Can you work these out from the model? Positions are in its coordinate system, mm. Round coordinates to 2 decimals unless told otherwise and drop trailing zeros. Order: outer loops, then holes, each group sorted by start corner. A loop starts at its lowest first (then second) coordinate and runs counter-clockwise, first axis right, second up. Notation, with made-up numbers: (83.25, -21) -> (115.25, -21) arc R20 ccw to (115.25, -16) -> close; hole circle Ø8 at (45, 1). An arc over 180 degrees is marked (long way). One line per item, written item: value.
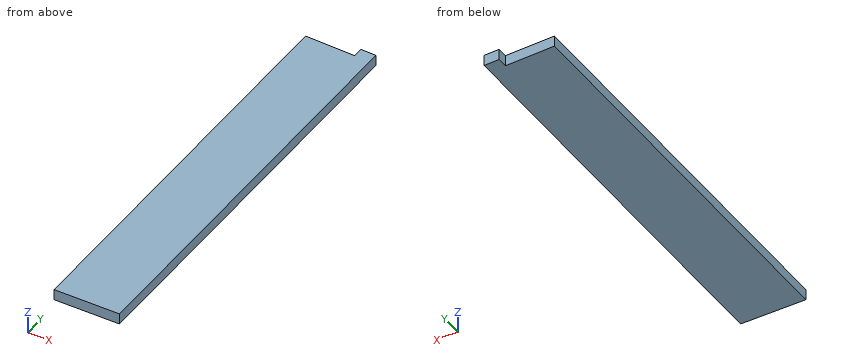
Autodesk Inventor part; units mm, degrees
ref_plane "YZ Plane" through (0, 0, 0) normal (1, 0, 0) x (0, 1, 0)
ref_plane "XZ Plane" through (0, 0, 0) normal (0, 1, 0) x (-1, 0, 0)
ref_plane "XY Plane" through (0, 0, 0) normal (0, 0, 1) x (1, 0, 0)
sketch "Sketch1" plane through (0, 0, 0) normal (0, 0, 1) x (1, 0, 0)
  line L0 (65.4735, 181.5397) -> (65.4735, -8.4603)
  line L1 (65.4735, -8.4603) -> (95.4735, -8.4603)
  line L2 (95.4735, -8.4603) -> (95.4735, 180.4921)
  line L3 (65.4735, 181.5397) -> (95.4735, 180.4921)
  line L4 (65.4735, 181.5397) -> (99.7821, 181.5397) construction
  line L5 (95.4735, 180.4921) -> (95.4735, 185.4921)
  line L6 (95.4735, 185.4921) -> (88.4735, 185.4921)
  line L7 (88.4735, 185.4921) -> (88.4735, 180.7366)
  line L8 (88.4735, 185.4921) -> (98.5031, 185.1419)
  line L9 (88.4735, 185.4921) -> (98.5092, 185.4921) construction
  point P0 (0, 0)
  point P1 (95.4735, 185.2477)
  dimension "d0" = 190
  dimension "d1" = 30
  dimension "d2" = 2
  dimension "d4" = 7
  dimension "d6" = 2
  dimension "d12" = 5
extrude "Extrusion1" add sketch "Sketch1" along normal blind 5 contours L3 L2 L1 L0 | L7 L8 L5 L3
properties part number "protostand"
Q1. Please list where these lines run through material, in increasing order: line 1 along Y through (x, z) = (88, 2.35); line 2 along Y through (x, z) = (79.5, 4.2).
Answers below:
line 1: -8.46 to 180.75
line 2: -8.46 to 181.05
Q2. I want a section at A-A on z = 1.2. List the corners of the cut face in (x, y) for me.
Answers below:
outline: (65.47, -8.46) -> (95.47, -8.46) -> (95.47, 185.25) -> (88.47, 185.49) -> (88.47, 180.74) -> (65.47, 181.54) -> close
Q3. Will this pin go through, and if not, where does the flat tip stop? pin 1 Ø8 at (x, y) = (78.5, 12) entering from -Z.
Answers below:
pin 1: z = 0
Q4. I want a section at C-C on x = 82. List the corners of the cut face in (y, z) for me.
Answers below:
outline: (-8.46, 0) -> (180.96, 0) -> (180.96, 5) -> (-8.46, 5) -> close
Q5. I want a section at B-B on x = 70. List the corners of the cut face in (y, z) for me.
Answers below:
outline: (-8.46, 0) -> (181.38, 0) -> (181.38, 5) -> (-8.46, 5) -> close
